```python
from build123d import *

# Parameters (mm, degrees)
F0_W     = 250
F0_H     = 350
F1_DEPTH = 100
F2_R     = 75
F3_DEPTH = 267
F4_W     = 70
F4_H     = 20
F5_DEPTH = 205


with BuildPart() as f1:
    # F0 (on Front) → F1 (new body)
    with BuildSketch(Plane.XZ):
        Rectangle(F0_W, F0_H)
    extrude(amount=F1_DEPTH)

    # F2 (on face) → F3 (cut)
    with BuildSketch(Plane.XZ.offset(100)):
        with Locations((-20.83086, -16.859313)):
            Circle(F2_R)
    extrude(amount=-F3_DEPTH, mode=Mode.SUBTRACT)

    # F4 (on face) → F5 (cut)
    with BuildSketch(Plane.XY.offset(175)):
        with Locations((29.123203, -60)):
            Rectangle(F4_W, F4_H)
    extrude(amount=-F5_DEPTH, mode=Mode.SUBTRACT)


solid = f1.part
```
Work out the finished part from the listing and answer in its coordinate system (mm). A direction names the side the tool comes from. Coordinates: 2 decimals unless noted, no trailing zeros. Loops run counter-clockwise (first coordinate to the right, second up) from the corner with the lowest first, then second, coordinate; pieces in that order, holes last.
1) Section D-D (y = -80) is taken. Give the vertices of the cut face in (x, z), plus the area to 3 significant figures.
Results:
outline: (-125, -175) - (125, -175) - (125, 175) - (-125, 175) - close; hole circle Ø150 at (-20.83, -16.86)
area: 69,800 mm2
2) Section C-C (z = 111) is taken. Give the vertices of the cut face in (x, y).
Results:
outline: (-125, -100) - (125, -100) - (125, 0) - (-125, 0) - close; hole (-5.88, -70) - (64.12, -70) - (64.12, -50) - (-5.88, -50) - close
3) Section B-B (z = -77.5) is taken. Give the vertices of the cut face in (x, y).
Results:
outline: (-125, -100) - (-64.96, -100) - (-64.96, 0) - (-125, 0) - close; (23.3, -100) - (125, -100) - (125, 0) - (23.3, 0) - close
4) A flat-ended cylindrical pin translates along its axis: pin 1 (5.5 mm diameter, centred on x = 61.5, y = -60, fed in from +Z). Find the tip coordinate at first contact, or state that the pin passes through.
Results:
pin 1: stops at z = 175
5) For a pull along X with two mould halves and no side action, classify faces 1 (the flat face through (125, -49, -2)), 2 (the flat face through (54, -100, 2)), 3 (the flat face through (29, -50, 97)) as +X half, -X half, draft (parallel to the pull), parting line (faces both ways), or undercut.
Results:
face 1: +X half
face 2: draft
face 3: undercut
6) Consider probe 1 along X at (y, z) = (-69, 64); probe 2 along Z at (x, y) = (-23.5, -71.5); probe 3 along Z at (x, y) = (19.5, -43). Determine where each line is inside the solid, lowest interval first.
Results:
probe 1: x = -125 to -5.88, 64.12 to 125
probe 2: z = -175 to -91.81, 58.09 to 175
probe 3: z = -175 to -80.09, 46.37 to 175
7) Section A-A (x = -70) is taken. Give the vertices of the cut face in (y, z).
Results:
outline: (-100, -175) - (0, -175) - (0, -73.49) - (-100, -73.49) - close; (-100, 39.77) - (0, 39.77) - (0, 175) - (-100, 175) - close
8) For faces 4 (the flat face through (54, 0, 2)), 5 (the flat face through (-5.877, -60, 117)), determine the directions among +Z, -Z, +X, -X, +Y, -Y from which every point of the face is accessible in a straight line to the end or side of a thin tool.
Results:
face 4: +Z, -Z, +X, -X, +Y
face 5: +Z
